Part print with two shaded views. Sizes in mm from the minimum x, y, z corner. A direction names the side the tool comes from. Round coordinates to 2 decimals unless told otherwise and drop trailing zeros. Write each loop counter-clockwise with the first axis right and the second up, starting at its lowest first coordinate (ties: lowest second). Pieces come first, ordered by that corner, then holes.
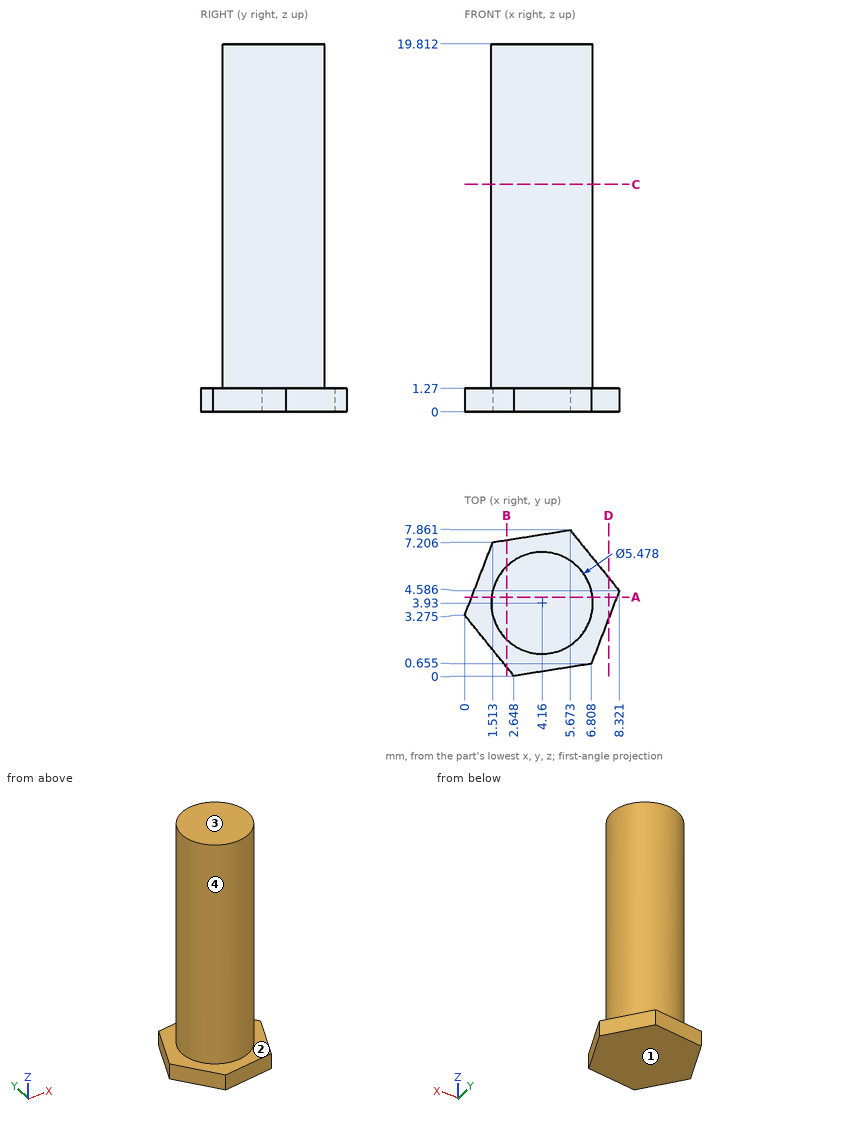
Q1. Wall check: L1, parallel to Z at x = 7, y = 2.75; L2, parallel to Y at x = 4.25, z = 17.5; L3, parallel to Y at x = 5.75, z = 3.75. Give the ranges that are in metal, low to high.
Values follow:
L1: z = 0 to 1.27
L2: y = 1.19 to 6.67
L3: y = 1.7 to 6.16
Q2. Cut at C-C on z = 12.25. Write the cut outline in (x, y), plus the area to 3 significant figures.
Values follow:
outline: circle Ø5.48 at (4.16, 3.93)
area: 23.6 mm2
Q3. Cut at B-B on x = 2.25. Write the cut outline in (y, z).
Values follow:
outline: (0.49, 0) - (7.32, 0) - (7.32, 1.27) - (5.89, 1.27) - (5.89, 19.81) - (1.97, 19.81) - (1.97, 1.27) - (0.49, 1.27) - close
Q4. Cut at A-A on y = 4.25. Write the cut outline in (x, z) (1 decimal), plus the area to 3 significant figures.
Values follow:
outline: (0.4, 0) - (8.2, 0) - (8.2, 1.3) - (6.9, 1.3) - (6.9, 19.8) - (1.4, 19.8) - (1.4, 1.3) - (0.4, 1.3) - close
area: 111 mm2
Q5. Drop flat-ended pins along their axis: pin 1 (4 mm diameter, centred on x = 2, y = 1, fed in from +Z); pin 2 (2 mm diameter, centred on x = 6, z = 9.5, fed in from -Y); pin 3 (4 mm diameter, centred on x = 7.5, z = 5.5, fed in from -Y); pin 4 (3 mm diameter, centred on y = 3.5, z = 15.5, fed in from -X). Give the stop position or say it passes through.
Values follow:
pin 1: stops at z = 19.81
pin 2: stops at y = 1.32
pin 3: stops at y = 1.54
pin 4: stops at x = 1.42
Q6. Cut at D-D on x = 7.75. Write the cut outline in (y, z).
Values follow:
outline: (3.1, 0) - (5.29, 0) - (5.29, 1.27) - (3.1, 1.27) - close
Q7. Mould opens along Y. For the marked faces 3 and 4 say: +Y half, -Y half, draft (parallel to the pull), parting line (faces both ways), or undercut.
Values follow:
face 3: draft
face 4: parting line
Q8. Which spindle directions (+Z, -Z, +X, -X, +Y, -Y) get a long thin tool onto all of the face, cutting with end or side? Do the marked faces 1 and 2. Say none if no direction does.
Values follow:
face 1: -Z, +X, -X, +Y, -Y
face 2: +Z
